Can you work these out from the drawing? Everything is in mm from the part's minimum corner. A direction names the side the tool comes from. Coordinates: 2 decimals unless noted, no trailing zeros. Order: outer loops, then holes, each group sorted by start corner. A loop starts at its lowest first (then second) coordinate and runs counter-clockwise, first axis right, second up. Notation, with made-up numbers: (52.5, 45) - (69.5, 45) arc R32 cw to (69.5, 74) - close; hole circle Ø1 at (82.5, 62). An arc over 180 degrees is marked (long way). Use a Markdown table: item, result. Add a question column.
(1) If I drill on L1, parallel to X at y = 12.5, z = 8.25; L2, parallel to Y at x = 9.5, z = 10.75, over which ranges is the centre line in solid material (lowest first)? Write a range as [from, to].
(2) On a 3-axis mill with a long thin cutter (end or side, diameter ignored), from which of +Z, -Z, +X, -X, +Y, -Y can I reach the whole of each face in a straight line? I mean the marked faces 4 and 5. Say none if no direction works.
(3) We'd pull the mould along X, two halves only. Please class the marked faces 1, 2 and 3: pulls with the +X half, pulls with the -X half, needs draft (parallel to the pull), parting line crosses it, or undercut.
(4) I want a section at B-B (z = 11). List the corners of the cut face in (x, y) for me, and give its area (3 significant figures).
(5) I want a section at A-A (x = 60). List the corners of the cut face in (y, z) for me.
(6) I want a section at D-D (x = 16). List the corners of the cut face in (y, z) for me.
(7) For pin 1 Ø6.5 at (y, z) = (60.5, 9) entering from -X; pin 2 Ø11 at (y, z) = (56, 7.5) entering from +X, each with a flat end and sliding along its axis, tell me the tip position at first contact or that it passes through.
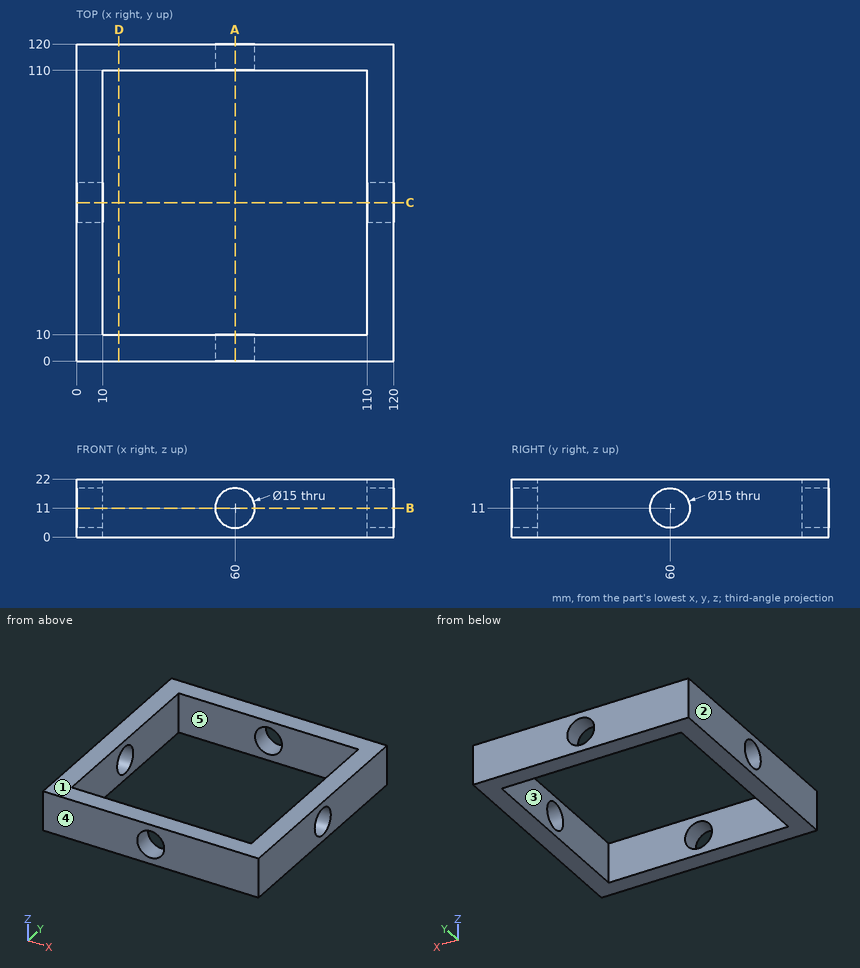
Answers follow:
| question | item | result |
|---|---|---|
| 1 | L1 | x = [0, 10], [110, 120] |
| 1 | L2 | y = [0, 52.5], [67.5, 120] |
| 2 | face 4 | +Z, -Z, +X, -X, -Y |
| 2 | face 5 | +Z, -Z |
| 3 | face 1 | needs draft |
| 3 | face 2 | pulls with the -X half |
| 3 | face 3 | undercut |
| 4 | outline | (0, 0) - (52.5, 0) - (52.5, 10) - (10, 10) - (10, 52.5) - (0, 52.5) - close; (0, 67.5) - (10, 67.5) - (10, 110) - (52.5, 110) - (52.5, 120) - (0, 120) - close; (67.5, 0) - (120, 0) - (120, 52.5) - (110, 52.5) - (110, 10) - (67.5, 10) - close; (67.5, 110) - (110, 110) - (110, 67.5) - (120, 67.5) - (120, 120) - (67.5, 120) - close |
| 4 | area | 3,800 mm² |
| 5 | outline | (0, 0) - (10, 0) - (10, 3.5) - (0, 3.5) - close; (0, 18.5) - (10, 18.5) - (10, 22) - (0, 22) - close; (110, 0) - (120, 0) - (120, 3.5) - (110, 3.5) - close; (110, 18.5) - (120, 18.5) - (120, 22) - (110, 22) - close |
| 6 | outline | (0, 0) - (10, 0) - (10, 22) - (0, 22) - close; (110, 0) - (120, 0) - (120, 22) - (110, 22) - close |
| 7 | pin 1 | passes through |
| 7 | pin 2 | stops at x = 120 |
